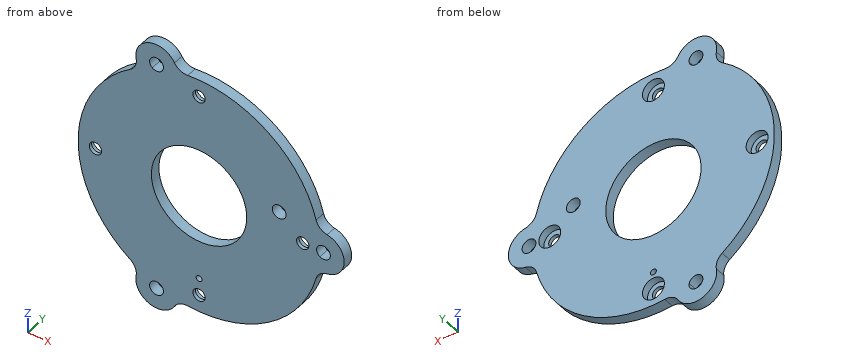
from build123d import *

# Parameters (mm, degrees)
SKETCH1_R                                      = 17.5
BOSS_EXTRUDE1_DEPTH                            = 1.5
CUT_EXTRUDE1_DEPTH                             = 25.794152536
CUT_EXTRUDE1_DEPTH_BACK                        = 25.794152536
SKETCH6_R                                      = 0.42
SKETCH6_R_2                                    = 1
CBORE_FOR_0_SOCKET_HEAD_CAP_SCREW1_D           = 1.778
CBORE_FOR_0_SOCKET_HEAD_CAP_SCREW1_CBORE_D     = 3.175
CBORE_FOR_0_SOCKET_HEAD_CAP_SCREW1_CBORE_DEPTH = 1.016
BOSS_EXTRUDE2_DEPTH                            = 1.5
FILLET1_R                                      = 2
CUT_EXTRUDE2_START                             = -10
SKETCH10_R                                     = 1
CUT_EXTRUDE2_DEPTH                             = 10
SKETCH11_R                                     = 6.9
CUT_EXTRUDE3_DEPTH                             = 10


with BuildPart() as part:
    # Sketch1 → Boss-Extrude1 (new body)
    with BuildSketch(Plane(origin=(0, 0, 0), x_dir=(1, 0, 0), z_dir=(0, 1, 0))):
        with Locations(Location((0, 0, 0), (0, 0, 270))):
            Circle(SKETCH1_R)
    extrude(amount=BOSS_EXTRUDE1_DEPTH)

    # Sketch6 → Cut-Extrude1 (cut, two sides: drawn at the far end of the back side and taken through both)
    with BuildSketch(Plane(origin=(0, 1.5, 0), x_dir=(1, 0, 0), z_dir=(0, 1, 0)).offset(-CUT_EXTRUDE1_DEPTH_BACK)):
        with Locations(Location((0, 12.5, 0), (0, 0, 270))):
            Circle(SKETCH6_R)
        with Locations(Location((11.591109915, -3.105828541, 0), (0, 0, 270))):
            Circle(SKETCH6_R_2)
    extrude(amount=CUT_EXTRUDE1_DEPTH + CUT_EXTRUDE1_DEPTH_BACK, mode=Mode.SUBTRACT)

    # CBORE for #0 Socket Head Cap Screw1 (through all)
    with Locations(Plane(origin=(0, 1.5, 0), x_dir=(1, 0, 0), z_dir=(0, 1, 0))):
        with Locations((0, 15), (-15, 0), (0, -15), (15, 0)):
            CounterBoreHole(CBORE_FOR_0_SOCKET_HEAD_CAP_SCREW1_D / 2, CBORE_FOR_0_SOCKET_HEAD_CAP_SCREW1_CBORE_D / 2, CBORE_FOR_0_SOCKET_HEAD_CAP_SCREW1_CBORE_DEPTH)

    # Sketch9 → Boss-Extrude2 (add)
    with BuildSketch(Plane.XZ):
        with BuildLine():
            ThreePointArc((-3.2615852, 17.702035532), (-7.18242301, 19.733545037), (-8.880129888, 15.657052506))
            Line((-8.880129888, 15.657052506), (-8.706640889, 15.180395398))
            ThreePointArc((-8.706640889, 15.180395398), (-7.758159345, 15.686330469), (-6.780403574, 16.133075571))
            ThreePointArc((-6.780403574, 16.133075571), (-6.498382723, 17.854159795), (-5.176050603, 16.717012297))
            ThreePointArc((-5.176050603, 16.717012297), (-4.139884011, 17.00327499), (-3.0880962, 17.225378424))
            Line((-3.0880962, 17.225378424), (-3.2615852, 17.702035532))
        make_face()
        with BuildLine():
            ThreePointArc((17.242752101, 2.989565186), (17.39377576, 1.925244093), (17.479166667, 0.853658385))
            ThreePointArc((17.479166667, 0.853658385), (19, 0), (17.479166667, -0.853658385))
            ThreePointArc((17.479166667, -0.853658385), (17.39377576, -1.925244093), (17.242752101, -2.989565186))
            Line((17.242752101, -2.989565186), (17.75, -2.989565186))
            ThreePointArc((17.75, -2.989565186), (21, 0), (17.75, 2.989565186))
            Line((17.75, 2.989565186), (17.242752101, 2.989565186))
        make_face()
        with BuildLine():
            ThreePointArc((-8.880129888, -15.657052506), (-7.18242301, -19.733545037), (-3.2615852, -17.702035532))
            Line((-3.2615852, -17.702035532), (-3.0880962, -17.225378424))
            ThreePointArc((-3.0880962, -17.225378424), (-4.139884011, -17.00327499), (-5.176050603, -16.717012297))
            ThreePointArc((-5.176050603, -16.717012297), (-6.498382723, -17.854159795), (-6.780403574, -16.133075571))
            ThreePointArc((-6.780403574, -16.133075571), (-7.758159345, -15.686330469), (-8.706640889, -15.180395398))
            Line((-8.706640889, -15.180395398), (-8.880129888, -15.657052506))
        make_face()
    extrude(amount=-BOSS_EXTRUDE2_DEPTH)

    # Fillet1
    fillet1_edges = [part.edges().sort_by_distance(p)[0] for p in [
        (17.242752101, 0.75, 2.989565186),
        (-3.0880962, 0.75, 17.225378424),
        (-8.706640889, 0.75, 15.180395398),
        (-8.706640889, 0.75, -15.180395398),
        (-3.0880962, 0.75, -17.225378424),
        (17.242752101, 0.75, -2.989565186),
    ]]
    fillet(fillet1_edges, radius=FILLET1_R)

    # Sketch10 → Cut-Extrude2 (cut)
    with BuildSketch(Plane(origin=(0, 1.5, 0), x_dir=(1, 0, 0), z_dir=(0, 1, 0)).offset(CUT_EXTRUDE2_START)):
        with Locations(Location((-6.15636258, 16.914467174, 0), (0, 0, 90))):
            Circle(SKETCH10_R)
        with Locations(Location((18, 0, 0), (0, 0, 90))):
            Circle(SKETCH10_R)
        with Locations(Location((-6.15636258, -16.914467174, 0), (0, 0, 90))):
            Circle(SKETCH10_R)
    extrude(amount=CUT_EXTRUDE2_DEPTH, mode=Mode.SUBTRACT)

    # Sketch11 → Cut-Extrude3 (cut)
    with BuildSketch(Plane(origin=(0, 1.5, 0), x_dir=(1, 0, 0), z_dir=(0, 1, 0))):
        with Locations(Location((0, 0, 0), (0, 0, 270))):
            Circle(SKETCH11_R)
    extrude(amount=-CUT_EXTRUDE3_DEPTH, mode=Mode.SUBTRACT)


solid = part.part
Model file for the job. Use its own axes, mm. Coordinates: 2 decimals unless noted, no trailing zeros. Order: outer loops, then holes, each group sorted by start corner. A loop starts at its lowest first (then second) coordinate and runs counter-clockwise, first axis right, second up. Notation, with made-up numbers: M 84.25,81.25 L 127.25,81.25 A15 cw 127.25,106.25 Z; hole C 72,76 d3. An arc over 180 degrees is marked long. Return JSON: item names as keys, results as strings.
1. Flat gauge pins, fed straight in: pin 1 (2.5 mm diameter, centred on x = 18, z = 0, fed in from +Y); pin 2 (3 mm diameter, centred on x = 0, z = -15, fed in from +Y). Where does each tip first touch, or does it go through?
Ans:
{"pin 1": "y = 1.5", "pin 2": "y = 0.48"}
2. Saw through at A-A (z = 0). Give the cut face in (x, y).
Ans:
{"outline": "M -17.5,0 L -15.89,0 L -15.89,0.48 L -16.59,0.48 L -16.59,1.5 L -17.5,1.5 Z; M -14.11,0 L -6.9,0 L -6.9,1.5 L -13.41,1.5 L -13.41,0.48 L -14.11,0.48 Z; M 6.9,0 L 14.11,0 L 14.11,0.48 L 13.41,0.48 L 13.41,1.5 L 6.9,1.5 Z; M 15.89,0 L 17,0 L 17,1.5 L 16.59,1.5 L 16.59,0.48 L 15.89,0.48 Z; M 19,0 L 21,0 L 21,1.5 L 19,1.5 Z"}
3. Saw through at D-D (y = 0.8). Give the number of separate pieces and of enclosed holes in the cut face, and give its area (3 significant figures).
Ans:
{"separate pieces": "1", "enclosed holes": "10", "area": "823 mm^2"}
4. Saw through at B-B (x = 4.5). Give the cut face in (y, z).
Ans:
{"outline": "M 0,-16.91 L 1.5,-16.91 L 1.5,-5.23 L 0,-5.23 Z; M 0,5.23 L 1.5,5.23 L 1.5,16.91 L 0,16.91 Z"}
5. Drill centre lines: probe 1 along X at (y, z) = (1.45, 5.5); probe 2 along Z at (x, y) = (3.5, 0.6); probe 3 along X at (y, z) = (1.25, -12.5). Where is each one in solid material? Low to high.
Ans:
{"probe 1": "-16.61 to -4.17, 4.17 to 16.61", "probe 2": "-17.15 to -5.95, 5.95 to 17.15", "probe 3": "-12.25 to -0.42, 0.42 to 12.25"}
6. Saw through at C-C (z = -5). Give the cut face in (x, y) (1 decimal).
Ans:
{"outline": "M -16.8,0 L -4.8,0 L -4.8,1.5 L -16.8,1.5 Z; M 4.8,0 L 16.8,0 L 16.8,1.5 L 4.8,1.5 Z"}
